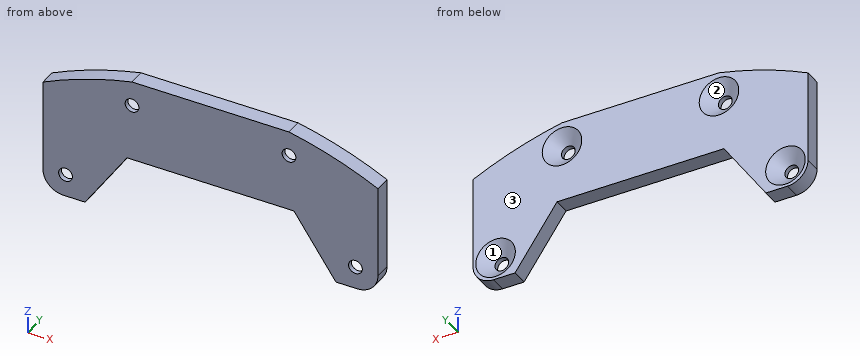
```python
from build123d import *

# Parameters (mm, degrees)
SKETCH1_R           = 1.35255
BOSS_EXTRUDE1_DEPTH = 3.175
CHAMFER2_SIZE       = 2.54635
CHAMFER2_SIZE2      = 2.213508285


with BuildPart() as part:
    # Sketch1 → Boss-Extrude1 (new body)
    with BuildSketch(Plane(origin=(0, 0, 0), x_dir=(1, 0, 0), z_dir=(0, 1, 0))):
        with BuildLine():
            Line((-24.73005605, 14.12875), (-16.454266742, 2.06375))
            Line((-16.454266742, 2.06375), (16.454266742, 2.06375))
            Line((16.454266742, 2.06375), (24.73005605, 14.12875))
            Line((24.73005605, 14.12875), (28.956, 14.12875))
            ThreePointArc((28.956, 14.12875), (31.829681959, 12.938431959), (33.02, 10.06475))
            Line((33.02, 10.06475), (33.02, -8.19025964))
            ThreePointArc((33.02, -8.19025964), (24.427649347, -11.694709026), (15.473036022, -14.12875))
            Line((15.473036022, -14.12875), (-15.473036022, -14.12875))
            ThreePointArc((-15.473036022, -14.12875), (-24.427649347, -11.694709026), (-33.02, -8.19025964))
            Line((-33.02, -8.19025964), (-33.02, 10.06475))
            ThreePointArc((-33.02, 10.06475), (-31.829681959, 12.938431959), (-28.956, 14.12875))
            Line((-28.956, 14.12875), (-24.73005605, 14.12875))
        make_face()
        with Locations((-28.575, 9.68375)):
            Circle(SKETCH1_R, mode=Mode.SUBTRACT)
        with Locations((-15.473036022, -9.2075)):
            Circle(SKETCH1_R, mode=Mode.SUBTRACT)
        with Locations((15.473036022, -9.2075)):
            Circle(SKETCH1_R, mode=Mode.SUBTRACT)
        with Locations((28.575, 9.68375)):
            Circle(SKETCH1_R, mode=Mode.SUBTRACT)
    extrude(amount=BOSS_EXTRUDE1_DEPTH)

    # Chamfer2
    chamfer2_edges = [part.edges().sort_by_distance(p)[0] for p in [
        (-16.825586022, 3.175, 9.2075),
        (-29.92755, 3.175, -9.68375),
        (14.120486022, 3.175, 9.2075),
        (27.22245, 3.175, -9.68375),
    ]]
    chamfer2_side = [part.faces().sort_by_distance(p)[0] for p in [
        (0, 3.175, 2.574836874),
    ]]
    chamfer(chamfer2_edges, length=CHAMFER2_SIZE, length2=CHAMFER2_SIZE2, reference=chamfer2_side[0])


solid = part.part
```
The model under review builds one solid part; all positions refer to its coordinate system, in mm. Face numbers are marked on the shaded views. Round coordinates to 2 decimals unless told otherwise and drop trailing zeros. Order: outer loops, then holes, each group sorted by start corner. A loop starts at its lowest first (then second) coordinate and runs counter-clockwise, first axis right, second up.
(1) Take a section at B-B, the plane z = -3.5. State the section outline as (x, y) points (3 decimals).
Working result:
outline: (-33.02, 0) - (-17.439, 0) - (-17.439, 3.175) - (-33.02, 3.175) - close; (17.439, 0) - (33.02, 0) - (33.02, 3.175) - (17.439, 3.175) - close
(2) Wall thickness on L1, parallel to X at y = 2.7, z = -11.25; L2, parallel to Z at x = -15.5, y = 0.8; L3, parallel to X at y = 2.9, z = 8.25: over which ranges is each line inside the solid? List them lowest first.
Working result:
L1: x = -32.84 to -31.54, -25.61 to -22.76, 22.76 to 25.61, 31.54 to 32.84
L2: z = -2.06 to 7.86, 10.56 to 14.12
L3: x = -32.9 to -18.93, -12.02 to 12.02, 18.93 to 32.9
(3) Take a section at A-A, the plane y = 2.55. State the section outline as (x, z) points (1 decimal).
Working result:
outline: (-33, -10.1) arc R4.1 ccw to (-29, -14.1) - (-24.7, -14.1) - (-16.5, -2.1) - (16.5, -2.1) - (24.7, -14.1) - (29, -14.1) arc R4.1 ccw to (33, -10.1) - (33, 8.2) arc R76.2 ccw to (15.5, 14.1) - (-15.5, 14.1) arc R76.2 ccw to (-33, 8.2) - close; hole circle Ø6.4 at (-28.6, -9.7); hole circle Ø6.4 at (-15.5, 9.2); hole circle Ø6.4 at (15.5, 9.2); hole circle Ø6.4 at (28.6, -9.7)
(4) For P1, Ø1, axis at x = 21.5, y = 0.5, coming from the +Z side; P2, Ø3, axis at x = 28.58, z = -9.68, coming from the +Y side, all flat-tipped, find the tip position at first contact; note any pin that passes through.
Working result:
P1: stops at z = 12.77
P2: stops at y = 1.1
(5) Mouldability with a two-part tool opening along X and no side actions: class the marked faces 1, 2 and 3 as released by +X, released by -X, zero draft, split by the parting line, or undercut.
Working result:
face 1: undercut
face 2: undercut
face 3: zero draft
(6) Take a section at C-C, the plane x = -23. State the section outline as (y, z) points (3 decimals), plus the area to 3 significant figures.
Working result:
outline: (0, -11.607) - (3.175, -11.607) - (3.175, 12.162) - (0, 12.162) - close
area: 75.5 mm2
(7) Take a section at D-D, the plane x = 2.5. State the section outline as (y, z) points (3 decimals), plus the area to 3 significant figures.
Working result:
outline: (0, -2.064) - (3.175, -2.064) - (3.175, 14.129) - (0, 14.129) - close
area: 51.4 mm2
